Build history of the part. All positions in model axes, mm. A direction names the side the tool comes from. Give positions to 0.01 mm unless a question says otherwise; leave off trailing zeros. Loops run counter-clockwise (first coordinate to the right, second up) from the corner with the lowest first, then second, coordinate; pieces in that order, holes last.
1) Two-plate mould, pull along X, no slides. Class faces 1 (the flat face through (24.137, 44.469, 4.93)), 2 (the flat face through (22.163, 12, 5)), 3 (the flat face through (14.694, 13, 5)), 4 (the flat face through (18, -2.386, 5)): +X half, -X half, draft (parallel to the pull), parting line (faces both ways), or undercut.
2) Band-saw the part on A-A on z = 7. List the corners of the cut face in (x, y).
3) Band-saw the part on B-B on y = 47. List the corners of the cut face in (x, z).
4) Band-saw the part on C-C on y = 23. List the corners of the cut face in (x, z), then the cut area to 3 significant figures.
5) Wall check: line 1 (X direction, y = 13, z = 2); line 2 (X direction, y = 44.5, z = 9.5); line 3 (Y direction, x = 6, z = 2.5). Give the ranges that are in metal, low to high.
6) Flat gauge pins, fed straight in: P1, Ø4, axis at y = 4, z = 5, coming from the +X side; P2, Ø12, axis at x = 11.5, y = 17.5, coming from the -Z side; P3, Ø3, axis at y = 25.5, z = 2.5, coming from the -X side. Where does each tip first touch, or does it go through?
7) Band-saw the part on D-D on x = 31. List the corners of the cut face in (y, z).
8) 3-axis set-ups, long thin cutter, end or side, ignore diameter. For faces 5 (the flat face through (13.22, 44.23, 4.93)), 6 (the flat face through (18, 32, 10)): which of +Z, -Z, +X, -X, +Y, -Y reach the whole face in a straight line?
```python
from build123d import *

# Parameters (mm, degrees)
F1_DEPTH = 10


with BuildPart() as f1:
    # F0 (on Top) → F1 (new body)
    with BuildSketch(Plane.XY):
        Polygon((21.119604, 31.836453), (18.428353, 27.614467), (18.428353, -2.385533), (22.162743, -2.385533), (22.162743, 27.614467), (38.288332, 52.912004), (34.553942, 52.912004), align=None)
        Polygon((2.302764, 52.912004), (18.428353, 27.614467), (21.119604, 31.836453), (18.601938, 35.786123), (7.685266, 52.912004), align=None)
        Polygon((18.428353, -2.385533), (18.428353, 27.614467), (2.302764, 52.912004), (-1.431626, 52.912004), (14.693964, 27.614467), (14.693964, -2.385533), align=None)
        Polygon((18.601938, 35.786123), (21.119604, 31.836453), (34.553942, 52.912004), (29.51861, 52.912004), align=None)
    extrude(amount=F1_DEPTH)


solid = f1.part
```
Findings below:
1. face 1: undercut
1. face 2: +X half
1. face 3: -X half
1. face 4: draft
2. outline: (-1.43, 52.91) - (14.69, 27.61) - (14.69, -2.39) - (22.16, -2.39) - (22.16, 27.61) - (38.29, 52.91) - (29.52, 52.91) - (18.6, 35.79) - (7.69, 52.91) - close
3. outline: (2.34, 0) - (11.45, 0) - (11.45, 10) - (2.34, 10) - close; (25.75, 0) - (34.52, 0) - (34.52, 10) - (25.75, 10) - close
4. outline: (14.69, 0) - (22.16, 0) - (22.16, 10) - (14.69, 10) - close
4. area: 74.7 mm2
5. line 1: x = 14.69 to 22.16
5. line 2: x = 3.93 to 13.05, 24.16 to 32.93
5. line 3: y = 41.25 to 52.91
6. P1: stops at x = 22.16
6. P2: stops at z = 0
6. P3: stops at x = 14.69
7. outline: (41.48, 0) - (52.91, 0) - (52.91, 10) - (41.48, 10) - close
8. face 5: +Z, -Z, +Y
8. face 6: +Z, +X, -X, +Y, -Y
